from build123d import *

# Parameters (mm, degrees)
F1_DEPTH = 25.4
F2_R     = 5.08


with BuildPart() as f1:
    # F0 (on Front) → F1 (new body)
    with BuildSketch(Plane.XZ):
        with BuildLine():
            Line((72.8656170726, 0.2934658736), (29.6668574194, 0.2934658736))
            ThreePointArc((29.6668574194, 0.2934658736), (0, 29.6683088726), (-29.6668574194, 0.2934658736))
            Line((-29.6668574194, 0.2934658736), (-62.2401205659, 0.2934658736))
            Line((-62.2401205659, 0.2934658736), (-62.2401205659, -63.2065341264))
            Line((-62.2401205659, -63.2065341264), (72.8656170726, -63.2065341264))
            Line((72.8656170726, -63.2065341264), (72.8656170726, 0.2934658736))
        make_face()
        with BuildLine():
            ThreePointArc((-22.5180355061, -6.0565341264), (0, 23.3183088726), (22.5180355061, -6.0565341264))
            Line((22.5180355061, -6.0565341264), (66.5156170726, -6.0565341264))
            Line((66.5156170726, -6.0565341264), (66.5156170726, -56.8565341264))
            Line((66.5156170726, -56.8565341264), (-55.8901205659, -56.8565341264))
            Line((-55.8901205659, -56.8565341264), (-55.8901205659, -6.0565341264))
            Line((-55.8901205659, -6.0565341264), (-22.5180355061, -6.0565341264))
        make_face(mode=Mode.SUBTRACT)
    extrude(amount=F1_DEPTH)

    # F2
    f2_edges = [f1.edges().sort_by_distance(p)[0] for p in [
        (51.266237, 0, 0.293466),
        (0, 0, 29.668309),
        (-45.953489, 0, 0.293466),
        (-62.240121, 0, -31.456534),
        (5.312748, 0, -63.206534),
        (72.865617, 0, -31.456534),
        (72.865617, -12.7, 0.293466),
        (-62.240121, -12.7, 0.293466),
        (29.666857, -12.7, 0.293466),
        (-29.666857, -12.7, 0.293466),
        (-45.953489, -25.4, 0.293466),
        (-62.240121, -12.7, -63.206534),
        (72.865617, -12.7, -63.206534),
        (51.266237, -25.4, 0.293466),
        (0, -25.4, 29.668309),
    ]]
    fillet(f2_edges, radius=F2_R)


solid = f1.part
For this review, take the finished solid that the model builds, in its own axes (mm). A direction names the side the tool comes from. Coordinates: 2 decimals unless noted, no trailing zeros. Order: outer loops, then holes, each group sorted by start corner. A loop starts at its lowest first (then second) coordinate and runs counter-clockwise, first axis right, second up. Notation, with made-up numbers: (-17.5, -19.5) - (11.5, -19.5) arc R29 ccw to (11.5, 5.5) - close; hole circle Ø8 at (55.25, 73). An arc over 180 degrees is marked (long way). Answer as CSV lines item,"result". Start each with the question number.
1) Draft analysis for pull direction Z (two halves, no side actions). For faces 5 (the flat face through (-62.24, -15, -31)), 6 (the cylindrical face through (-30.99, -12.807, 1.547)), 7 (the flat face through (6, -13, -56.857)), 8 (the flat face through (-39, -13, -6.057)), state which applies: +Z half, -Z half, draft (parallel to the pull), parting line (faces both ways), or undercut.
2) Add section C-C (y = -14). State the section outline as (x, z) points, then the cut area to 3 significant figures.
3) Insertion check: P1, Ø3, axis at y = -18, z = -4, coming from the -X side; P2, Ø12, axis at x = 49.5, y = -9.5, coming from the +Z side; P3, Ø8, axis at x = 7, y = -18, coming from the +Z side; P4, Ø5, axis at x = 35.5, y = -17, coming from the +Z side. Each pin has a flat end and moves straight along its axis. Give the tip position at first contact, or say it passes through.
4) Add section B-B (x = 0). State the section outline as (y, z) points.
5) Add section A-A (z = -51). State the section outline as (x, y) points, then the cut area to 3 significant figures.
6) Add section D-D (y = -22). State the section outline as (x, z) points, then the cut area to 3 significant figures.
7) To check wall thickness, follow line 1 along X through (y, z) = (-12.25, -34); line 2 along Z through (x, y) = (58, -8.25); line 3 along Z through (x, y) = (0, -16.25). State the ranges of each line that lie inside material, in increasing order. Write a range as [from, to].
8) Machinability: for faces 1 (the cylindrical face through (53.328, -23.872, -1.155)), 2 (the cylindrical face through (-48.481, -23.872, -1.155)), 3 (the flat face through (51, -13, 0.293)), 4 (the flat face through (-55.89, -13, -32)), which of the approach directions +Z, -Z, +X, -X, +Y, -Y give a long, thin tool a straight path to every point of the face, cutting with its end or side? Answer none if there is none.
Result:
1,face 5,"draft"
1,face 6,"+Z half"
1,face 7,"undercut"
1,face 8,"undercut"
2,outline,"(-62.24, -58.13) arc R5.08 ccw to (-57.16, -63.21) - (67.79, -63.21) arc R5.08 ccw to (72.87, -58.13) - (72.87, -4.79) arc R5.08 ccw to (67.79, 0.29) - (34.33, 0.29) arc R5.08 cw to (29.31, 4.59) arc R29.67 ccw to (-29.31, 4.59) arc R5.08 cw to (-34.33, 0.29) - (-57.16, 0.29) arc R5.08 ccw to (-62.24, -4.79) - close; hole (-55.89, -56.86) - (66.52, -56.86) - (66.52, -6.06) - (22.52, -6.06) arc R23.32 ccw (long way) to (-22.52, -6.06) - (-55.89, -6.06) - close"
2,area,"2,580 mm^2"
3,P1,"x = -62.24"
3,P2,"z = 0.29"
3,P3,"z = 29.52"
3,P4,"z = 0.47"
4,outline,"(-25.4, -63.21) - (-5.08, -63.21) arc R5.08 ccw to (0, -58.13) - (0, -56.86) - (-25.4, -56.86) - close; (-25.4, 23.32) - (0, 23.32) - (0, 24.59) arc R5.08 ccw to (-5.08, 29.67) - (-20.32, 29.67) arc R5.08 ccw to (-25.4, 24.59) - close"
5,outline,"(-62.24, -25.4) - (-55.89, -25.4) - (-55.89, 0) - (-57.16, 0) arc R5.08 ccw to (-62.24, -5.08) - close; (66.52, -25.4) - (72.87, -25.4) - (72.87, -5.08) arc R5.08 ccw to (67.79, 0) - (66.52, 0) - close"
5,area,"312 mm^2"
6,outline,"(-62.24, -58.13) arc R5.08 ccw to (-57.16, -63.21) - (67.79, -63.21) arc R5.08 ccw to (72.87, -58.13) - (72.87, -4.79) arc R5.08 ccw to (69.47, 0.01) - (34.33, 0.01) arc R5.37 cw to (29.03, 4.54) arc R29.38 ccw to (-29.03, 4.54) arc R5.37 cw to (-34.33, 0.01) - (-58.84, 0.01) arc R5.08 ccw to (-62.24, -4.79) - close; hole (-55.89, -56.86) - (66.52, -56.86) - (66.52, -6.06) - (22.52, -6.06) arc R23.32 ccw (long way) to (-22.52, -6.06) - (-55.89, -6.06) - close"
6,area,"2,530 mm^2"
7,line 1,"[-62.24, -55.89], [66.52, 72.87]"
7,line 2,"[-63.21, -56.86], [-6.06, 0.29]"
7,line 3,"[-63.21, -56.86], [23.32, 29.67]"
8,face 1,"+Z, +X, -Y"
8,face 2,"+Z, -X, -Y"
8,face 3,"+Z, +X, +Y, -Y"
8,face 4,"+Y, -Y"
